For this review, take the finished solid that the model builds, in its own axes (mm). A direction names the side the tool comes from. Round coordinates to 2 decimals unless told otherwise and drop trailing zeros. Loops run counter-clockwise (first coordinate to the right, second up) from the corner with the lowest first, then second, coordinate; pieces in that order, holes last.
1) Tool access review of faces 5 (the flat face through (-1.588, -8, 6)), 6 (the flat face through (-7, 4.331, 8)): name each direction out of +Z, -Z, +X, -X, +Y, -Y from which nothing blocks a thin tool from reaching the whole face with its end or side.
2) Take a section at A-A (y = 10.5). State the section outline as (x, z) points, then the cut area to 3 significant figures.
3) Insertion check: pin 1 (1.9 mm diameter, centred on x = 9.5, z = 7.5, fed in from +Y); pin 2 (1 mm diameter, centred on y = -14, z = 10, fed in from +X); pin 3 (5 mm diameter, centred on x = -6.5, z = 8, fed in from -Y). Each pin has a flat end and moves straight along its axis. Give the tip position at first contact, or say it passes through.
4) Mouldability with a two-part tool opening along X and no side actions: class faces 1 (the flat face through (3.97, 0.27, 12.58)), 2 (the cylindrical face through (18.17, 5.72, 5.82)), 3 (the flat face through (-9, 1.588, 3)), 4 (the flat face through (0, 0, 9)) as pulls with the +X half, pulls with the -X half, needs draft (parallel to the pull), parting line crosses it, or undercut.
5) Take a section at C-C (x = -13.5). State the section outline as (y, z) points, then the cut area to 3 significant figures.
6) Take a section at B-B (z = 7). Give the number of separate pieces and of enclosed holes in the cut face, then the cut area to 3 significant figures.
7) Wall thickness on L1, parallel to Y at x = 0, z = 2.25; L2, parallel to X at y = -1, z = 8; L3, parallel to Z at x = -0.5, y = -0.5: over which ranges is each line inside the solid? List them lowest first.
```python
from build123d import *

# Parameters (mm, degrees)
F0_R          = 19.05
F1_DEPTH      = 25.4
F3_DEPTH      = 19.051
F3_DEPTH_BACK = 19.051
F5_DEPTH      = 15.241
F8_DEPTH      = 10.16


with BuildPart() as f1:
    # F0 (on Top) → F1 (new body)
    with BuildSketch(Plane.XY):
        Circle(F0_R)
    extrude(amount=F1_DEPTH)

    # F2 (on Front) → F3 (cut, two sides)
    with BuildSketch(Plane.XZ) as f3_sk:
        Polygon((-19.05, 25.4), (-19.05, 8.521942), (19.05, 15.24), (19.05, 25.4), align=None)
    extrude(amount=F3_DEPTH, mode=Mode.SUBTRACT)
    extrude(f3_sk.sketch, amount=-F3_DEPTH_BACK, mode=Mode.SUBTRACT)

    # F4 (on Top) → F5 (cut, through all)
    with BuildSketch(Plane.XY):
        with BuildLine():
            Line((-1.5875, -4.953), (-1.5875, -11.303))
            ThreePointArc((-1.5875, -11.303), (0, -12.8905), (1.5875, -11.303))
            Line((1.5875, -11.303), (1.5875, -4.953))
            ThreePointArc((1.5875, -4.953), (0, -3.3655), (-1.5875, -4.953))
        make_face()
        with BuildLine():
            Line((-1.5875, 11.303), (-1.5875, 4.953))
            ThreePointArc((-1.5875, 4.953), (0, 3.3655), (1.5875, 4.953))
            Line((1.5875, 4.953), (1.5875, 11.303))
            ThreePointArc((1.5875, 11.303), (0, 12.8905), (-1.5875, 11.303))
        make_face()
        with BuildLine():
            Line((12.573, 1.5875), (6.223, 1.5875))
            ThreePointArc((6.223, 1.5875), (4.6355, 0), (6.223, -1.5875))
            Line((6.223, -1.5875), (12.573, -1.5875))
            ThreePointArc((12.573, -1.5875), (14.1605, 0), (12.573, 1.5875))
        make_face()
        with BuildLine():
            Line((-12.573, -1.5875), (-6.223, -1.5875))
            ThreePointArc((-6.223, -1.5875), (-4.6355, 0), (-6.223, 1.5875))
            Line((-6.223, 1.5875), (-12.573, 1.5875))
            ThreePointArc((-12.573, 1.5875), (-14.1605, 0), (-12.573, -1.5875))
        make_face()
    extrude(amount=F5_DEPTH, mode=Mode.SUBTRACT)

    # F7 (on offset) → F8 (cut)
    with BuildSketch(Plane.XY.offset(15.24)):
        with BuildLine():
            ThreePointArc((-12.573, 4.3307), (-16.9037, 0), (-12.573, -4.3307))
            Line((-12.573, -4.3307), (-6.223, -4.3307))
            Line((-6.223, -4.3307), (0, -4.3307))
            Line((0, -4.3307), (0, 4.3307))
            Line((0, 4.3307), (-6.223, 4.3307))
            Line((-6.223, 4.3307), (-12.573, 4.3307))
        make_face()
    extrude(amount=-F8_DEPTH, mode=Mode.SUBTRACT)


solid = f1.part
```
Response:
1. face 5: +Z, -Z
1. face 6: +Z
2. outline: (-15.9, 0) - (-1.59, 0) - (-1.59, 11.6) - (-15.9, 9.08) - close; (1.59, 0) - (15.9, 0) - (15.9, 14.68) - (1.59, 12.16) - close
2. area: 340 mm2
3. pin 1: stops at y = 17.02
3. pin 2: stops at x = 13.44
3. pin 3: stops at y = -18.63
4. face 1: pulls with the -X half
4. face 2: parting line crosses it
4. face 3: undercut
4. face 4: undercut
5. outline: (-13.44, 0) - (-1.29, 0) - (-1.29, 5.08) - (-4.23, 5.08) - (-4.23, 9.5) - (-13.44, 9.5) - close; (1.29, 0) - (13.44, 0) - (13.44, 9.5) - (4.23, 9.5) - (4.23, 5.08) - (1.29, 5.08) - close
5. area: 205 mm2
6. separate pieces: 1
6. enclosed holes: 2
6. area: 920 mm2
7. L1: y = -19.05 to -12.89, -3.37 to 3.37, 12.89 to 19.05
7. L2: x = -19.02 to -16.79, 0 to 4.99, 13.81 to 19.02
7. L3: z = 0 to 5.08
